```python
from build123d import *

# Parameters (mm, degrees)
F1_DEPTH = 114.935
F3_DEPTH = 92.075
F0_W     = 280
F0_H     = 40
F4_DEPTH = 195.58
F2_W     = 279.510707
F2_H     = 37.612499
F5_DEPTH = 133.35


with BuildPart() as f1:
    # F0 (on Right) → F1 (new body)
    with BuildSketch(Plane.YZ):
        Polygon((-129.108052, 51.825723), (-129.108052, -2.174277), (150.891948, -2.174277), (150.891948, 121.825723), (70.891948, 201.825723), (20.891948, 201.825723), align=None)
    extrude(amount=F1_DEPTH)

    # F0 (on Right) → F3 (join)
    with BuildSketch(Plane.YZ):
        Polygon((-129.108052, 51.825723), (-129.108052, -2.174277), (150.891948, -2.174277), (150.891948, 121.825723), (70.891948, 201.825723), (20.891948, 201.825723), align=None)
    extrude(amount=-F3_DEPTH)

    # F0 (on Right) → F4 (join)
    with BuildSketch(Plane.YZ):
        with Locations((10.891948, -22.174277)):
            Rectangle(F0_W, F0_H)
    extrude(amount=F4_DEPTH)

    # F2 (on Right) → F5 (join)
    with BuildSketch(Plane.YZ):
        with Locations((11.174976, -23.099343)):
            Rectangle(F2_W, F2_H)
    extrude(amount=-F5_DEPTH)


solid = f1.part
```
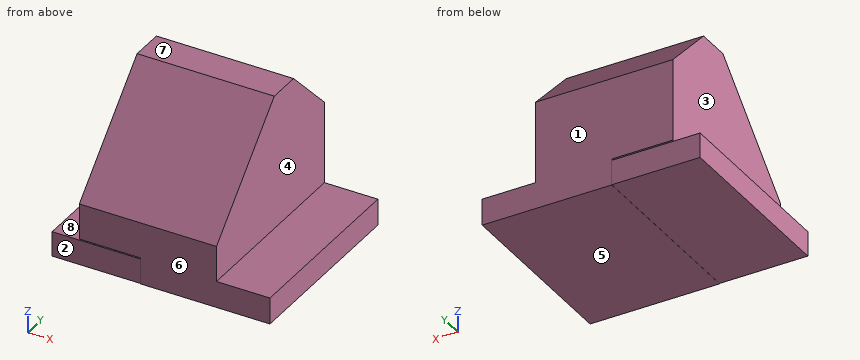
Work out the finished part from the listing and answer in its coordinate system (mm). Face numbers are marked on the shaded views. A direction names the side the tool comes from. Round coordinates to 2 decimals unless told otherwise and drop trailing zeros. Write each loop counter-clockwise with the first axis right and the second up, starting at its lowest first coordinate (ties: lowest second). Pieces come first, ordered by that corner, then holes. Notation, with made-up numbers: (32, -39.75) - (68, -39.75) arc R27 ccw to (68, -14.75) - close; hole circle Ø1 at (-12, 2.5). An arc over 180 degrees is marked (long way). Return JSON: item names as keys, results as strings. Group by question number.
Q1. The part is cut by section C-C on x = 93. Write down the section's boundary in (y, z), then the cut area to 3 significant figures.
Q2. The part is cut by section D-D on z = 79. Write down the section's boundary in (x, y) (3 decimals), then the cut area to 3 significant figures.
Q3. Each of these flat-tipped pins is pushed along its axis until it touches: pin 1 Ø5 at (x, z) = (-50.5, 128) entering from -Y; pin 2 Ø10 at (x, y) = (23, 107) entering from +Z; pin 3 Ø8 at (y, z) = (122.5, 51.5) entering from +X (3 decimals). Where does it stop, or does it pass through?
Q4. The mould has two halves that part along Z. Classify the marked faces 5, 6, 7 and 8: released by +Z, released by -Z, zero draft, split by the parting line, or undercut.
Q5. Find the intervals of material crossed by L1, parallel to Z at x = -5, y = 57.5; L2, parallel to Y at x = -31, z = 39.5; L3, parallel to X at y = 32.5, z = 11 (3 decimals), in increasing order.
Q6. The part is cut by section A-A on x = -62. Write down the section's boundary in (y, z), then the cut area to 3 significant figures.
Q7. For the marked faces 1, 2, 3 and 4, determine the directions among +Z, -Z, +X, -X, +Y, -Y from which every point of the face is accessible in a straight line to the end or side of a thin tool.
Q8. The part is cut by section B-B on y = 27. Write down the section's boundary in (x, z) (3 decimals), then the cut area to 3 significant figures.
Solved:
{
 "1": {"outline": "(-129.11, -42.17) - (150.89, -42.17) - (150.89, 121.83) - (70.89, 201.83) - (20.89, 201.83) - (-129.11, 51.83) - close", "area": "53,900 mm²"},
 "2": {"outline": "(-92.075, -101.934) - (114.935, -101.934) - (114.935, 150.892) - (-92.075, 150.892) - close", "area": "52,300 mm²"},
 "3": {"pin 1": "y = -55.43", "pin 2": "z = 170.72", "pin 3": "x = 114.935"},
 "4": {"face 5": "released by -Z", "face 6": "zero draft", "face 7": "released by +Z", "face 8": "undercut"},
 "5": {"L1": "-41.91 to -4.29, -2.17 to 201.83", "L2": "-129.11 to 150.89", "L3": "-92.075 to 114.935"},
 "6": {"outline": "(-129.11, -2.17) - (150.89, -2.17) - (150.89, 121.83) - (70.89, 201.83) - (20.89, 201.83) - (-129.11, 51.83) - close; (-128.58, -41.91) - (150.93, -41.91) - (150.93, -4.29) - (-128.58, -4.29) - close", "area": "53,200 mm²"},
 "7": {"face 1": "+Z, -Z, +X, -X, +Y", "face 2": "-Z, -X, -Y", "face 3": "+Z, -X, +Y, -Y", "face 4": "+Z, +X, +Y, -Y"},
 "8": {"outline": "(-133.35, -41.906) - (0, -41.906) - (0, -42.174) - (195.58, -42.174) - (195.58, -2.174) - (114.935, -2.174) - (114.935, 201.826) - (-92.075, 201.826) - (-92.075, -2.174) - (0, -2.174) - (0, -4.293) - (-133.35, -4.293) - close", "area": "55,100 mm²"}
}
